The listing builds one solid part. Answer for the finished solid, in the listing's coordinates (mm). Face numbers are marked on the shaded views. Coordinates: 2 decimals unless noted, no trailing zeros. Write each loop counter-clockwise with the first axis right and the second up, starting at its lowest first coordinate (ties: lowest second). Pieces come first, ordered by that corner, then holes. Notation, with made-up numbers: M 2.5,56.5 L 59.5,56.5 A27 cw 59.5,75.5 Z; hole C 22.25,47.25 d1. An arc over 180 degrees is marked long. Put each result on its own line as item: value. Start each with the question number.
```python
from build123d import *

# Parameters (mm, degrees)
SKETCH1_W           = 211.1375
SKETCH1_H           = 35.56
BOSS_EXTRUDE1_DEPTH = 9.525
SKETCH6_R           = 12.192
BOSS_EXTRUDE4_DEPTH = 6.35
BOSS_EXTRUDE5_DEPTH = 3.175
LPATTERN1_COUNT     = 22
LPATTERN1_PITCH     = 9.525


with BuildPart() as part:
    # Sketch1 → Boss-Extrude1 (new body)
    with BuildSketch(Plane(origin=(0, 0, 0), x_dir=(1, 0, 0), z_dir=(0, 1, 0))):
        with Locations((-105.56875, 17.78)):
            Rectangle(SKETCH1_W, SKETCH1_H)
    extrude(amount=BOSS_EXTRUDE1_DEPTH)

    # Sketch6 → Boss-Extrude4 (add)
    with BuildSketch(Plane(origin=(0, 0, 0), x_dir=(-1, 0, 0), z_dir=(0, -1, 0))):
        with Locations((105.56875, 17.78)):
            Circle(SKETCH6_R)
        with Locations((36.79825, 17.78)):
            Circle(SKETCH6_R)
        with Locations((174.33925, 17.78)):
            Circle(SKETCH6_R)
    extrude(amount=BOSS_EXTRUDE4_DEPTH)

    # Sketch9 → Boss-Extrude5 (add)
    with BuildSketch(Plane.ZY.offset(204.7875)):
        Polygon((-35.56, 9.525), (0, 9.525), (-8.89, 34.417), align=None)
    boss_extrude5 = extrude(amount=-BOSS_EXTRUDE5_DEPTH)

    # LPattern1: Boss-Extrude5 ×22
    with Locations(*[(i * LPATTERN1_PITCH, 0, 0) for i in range(1, LPATTERN1_COUNT)]):
        add(boss_extrude5)


solid = part.part
```
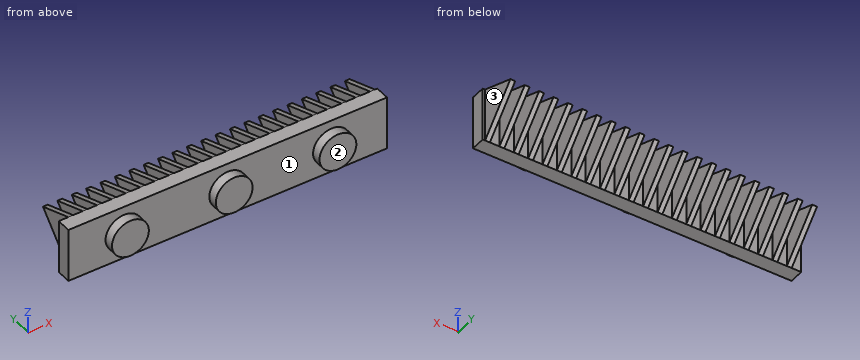
1) Straight lines are drawn through the part: probe 1 along X at (y, z) = (-1.5, -12.5); probe 2 along Y at (x, z) = (-86, -6) (3 decimals); probe 3 along Y at (x, z) = (-169.5, -11.5) (3 decimals). For each, find the intervals that lie inside material, in ascending order.
2) A cutting plane is placed at B-B on y = 19. State how many separate pieces and enclosed holes the cut face has, then the cut area to 3 significant figures.
3) Determine the mould class of the marked faces 1, 2 and 3 for opening direction X: +X half, -X half, draft (parallel to the pull), parting line (faces both ways), or undercut.
4) A cutting plane is placed at A-A on x = -159. Write down the section's boundary in (y, z) (3 decimals), then the cut area to 3 significant figures.
5) Given pin 1 Ø7.5 at (y, z) = (26, -21) entering from +X; pin 2 Ø1.9 at (x, z) = (-25.5, -15.5) entering from +Y (3 decimals); pin 3 Ø7.5 at (y, z) = (18.5, -11) entering from -X; pin 4 Ø4 at (y, z) = (-0.5, -29.5) entering from -X, each flat-ended and moving along its own axis, determine where each tip first touches the part or whether it passes through.
Answers follow:
1. probe 1: x = -185.33 to -163.35, -116.56 to -94.58, -47.79 to -25.81
1. probe 2: y = 0 to 9.525
1. probe 3: y = -6.35 to 9.525
2. separate pieces: 22
2. enclosed holes: 0
2. area: 1,540 mm²
3. face 1: undercut
3. face 2: draft
3. face 3: +X half
4. outline: M 0,-35.56 L 9.525,-35.56 L 9.525,0 L 0,0 Z
4. area: 339 mm²
5. pin 1: stops at x = -1.59
5. pin 2: stops at y = 9.525
5. pin 3: stops at x = -204.79
5. pin 4: stops at x = -211.14
